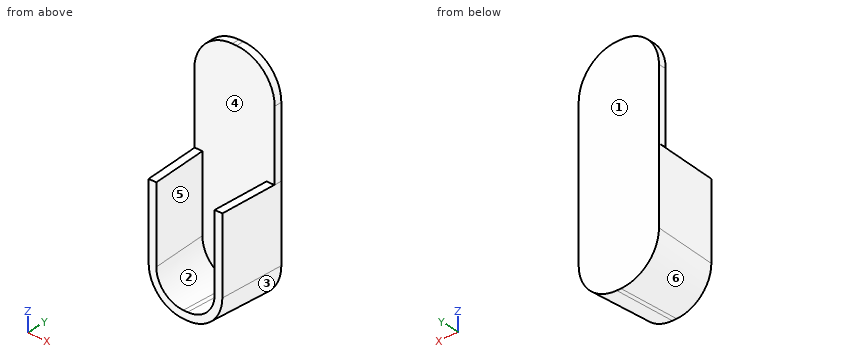
from build123d import *

# Parameters (mm, degrees)
F1_DEPTH = 15
F1_TAPER = 3.0006
F2_T     = -1.8
F3_W     = 16.786262393
F3_H     = 17.0369902626
F4_DEPTH = 28
F6_DEPTH = 1.8


# Not quite as in the source:
# - ends of sketch curves that miss each other by under 0.0002 mm in the source are joined


with BuildPart() as f1:
    # F0 (on Front) → F1 (new body)
    with BuildSketch(Plane.XZ):
        with BuildLine():
            Line((0.5, 19.5), (-0.5, 19.5))
            ThreePointArc((-0.5, 19.5), (-6.8639610307, 16.8639610307), (-9.5, 10.5))
            Line((-9.5, 10.5), (-9.5, -10.5))
            ThreePointArc((-9.5, -10.5), (-6.8639610307, -16.8639610307), (-0.5, -19.5))
            Line((-0.5, -19.5), (0.5, -19.5))
            ThreePointArc((0.5, -19.5), (6.8639610307, -16.8639610307), (9.5, -10.5))
            Line((9.5, -10.5), (9.5, 10.5))
            ThreePointArc((9.5, 10.5), (6.8639610307, 16.8639610307), (0.5, 19.5))
        make_face()
    extrude(amount=F1_DEPTH, taper=F1_TAPER)

    # F2
    f2_openings = [f1.faces().sort_by_distance(p)[0] for p in [
        (0, 0, 0),
        (0, -15, 0),
    ]]
    offset(amount=F2_T, openings=f2_openings)

    # F3 (on Right) → F4 (cut, symmetric)
    with BuildSketch(Plane.YZ):
        with Locations((-8.3931311965, 15.8226261847)):
            Rectangle(F3_W, F3_H)
    extrude(amount=F4_DEPTH, both=True, mode=Mode.SUBTRACT)

    # F5 (on face) → F6 (join)
    with BuildSketch(Plane(origin=(0, 0, 0), x_dir=(-1, 0, 0), z_dir=(0, 1, 0))):
        with BuildLine():
            Line((0.5000003055, 32.8999999631), (-0.4999996945, 32.8999999631))
            ThreePointArc((-0.4999996945, 32.8999999631), (-6.8639607252, 30.2639609938), (-9.4999996945, 23.8999999631))
            Line((-9.4999996945, 23.8999999631), (-9.4999998419, 7.3041310534))
            Line((-9.4999998419, 7.3041310534), (-7.6975287879, 7.3041310534))
            Line((-7.6975287879, 7.3041310534), (-7.6975287879, -10.5))
            ThreePointArc((-7.6975287879, -10.5), (-5.5894214137, -15.5894214137), (-0.5, -17.6975287879))
            Line((-0.5, -17.6975287879), (0.5, -17.6975287879))
            ThreePointArc((0.5, -17.6975287879), (5.5894214137, -15.5894214137), (7.6975287879, -10.5))
            Line((7.6975287879, -10.5), (7.6975287879, 7.3041310534))
            Line((7.6975287879, 7.3041310534), (9.5, 7.3041310534))
            Line((9.5, 7.3041310534), (9.5000003055, 23.8999999631))
            ThreePointArc((9.5000003055, 23.8999999631), (6.8639613362, 30.2639609938), (0.5000003055, 32.8999999631))
        make_face()
    extrude(amount=-F6_DEPTH)


solid = f1.part
Check sheet for the modelled part. Datum: model origin and axes. Units: mm. Face numbers are marked on the shaded views. A direction names the side the tool comes from. Give positions to 0.01 mm unless a question says otherwise; leave off trailing zeros. Order: outer loops, then holes, each group sorted by start corner. A loop starts at its lowest first (then second) coordinate and runs counter-clockwise, first axis right, second up. Notation, with made-up numbers: M 12.5,78.25 L 18.5,78.25 A14 ccw 18.5,103.25 Z; hole C 58.5,30.5 d1. An arc over 180 degrees is marked long. Answer as CSV lines item,"result". Start each with the question number.
Item 1: Tool access check on the marked faces 1 and 2. Record the directions out of +Z, -Z, +X, -X, +Y, -Y that give a thin tool (end or side, any length) a straight path to the whole face; none if there is none.
Item 2: Cross-section at A-A on z = 26. Enter the section's corners in (x, y), plus the area to 3 significant figures.
Item 3: Thickness scan on line 1 (Y direction, x = 5.5, z = 24); line 2 (X direction, y = -11.75, z = 6.5); line 3 (X direction, y = -14, z = 1). Record the ranges inside material, lowest first. Write a range as [from, to].
Item 4: Mould release check, pull along X, two halves, no side actions. Record for the marked faces 3, 4, 5 and 6: +X half, -X half, draft (parallel to the pull), parting line (faces both ways), or undercut.
Item 5: Gauge pin test, flat ends, axial feed: P1, Ø1, axis at y = -7.5, z = -5.5, coming from the -X side; P2, Ø6, axis at y = -8.5, z = 11.5, coming from the -X side; P3, Ø2, axis at y = -2, z = 1.5, coming from the +X side; P4, Ø6, axis at x = -0.5, y = -10.5, coming from the +Z side. Record the tip position at first contact, or that the pin passes through.
Established:
1,face 1,"+Z, -Z, +X, -X, +Y"
1,face 2,"+Z"
2,outline,"M -9.25,-1.8 L 9.25,-1.8 L 9.25,0 L -9.25,0 Z"
2,area,"33.3 mm^2"
3,line 1,"y = [-1.8, 0]"
3,line 2,"x = [-8.88, -7.08], [7.08, 8.88]"
3,line 3,"x = [-8.77, -6.96], [6.96, 8.77]"
4,face 3,"+X half"
4,face 4,"undercut"
4,face 5,"undercut"
4,face 6,"-X half"
5,P1,"stops at x = -9.13"
5,P2,"passes through"
5,P3,"stops at x = 9.45"
5,P4,"stops at z = -16.42"
